The listing builds one solid part. Answer for the finished solid, in the listing's coordinates (mm). A direction names the side the tool comes from. Round coordinates to 2 decimals unless told otherwise and drop trailing zeros. Loops run counter-clockwise (first coordinate to the right, second up) from the corner with the lowest first, then second, coordinate; pieces in that order, holes last. Notation, with made-up numbers: (81, 66.25) -> (136, 66.25) arc R30 ccw to (136, 88.25) -> close; hole circle Ø9 at (-26.75, 70.25). An arc over 180 degrees is marked (long way). Answer in a Markdown table with one row per item. Add a question column.
Autodesk Inventor part; units mm, degrees
ref_plane "YZ Plane" through (0, 0, 0) normal (1, 0, 0) x (0, 1, 0)
ref_plane "XZ Plane" through (0, 0, 0) normal (0, 1, 0) x (-1, 0, 0)
ref_plane "XY Plane" through (0, 0, 0) normal (0, 0, 1) x (1, 0, 0)
sketch "Sketch1" plane through (0, 0, 0) normal (0, 0, 1) x (1, 0, 0)
  line L0 (-85, 50) -> (85, 50)
  line L1 (85, 50) -> (85, -50)
  line L2 (85, -50) -> (-85, -50)
  line L3 (-85, -50) -> (-85, 50)
  line L4 (-85, 50) -> (85, -50) construction
  line L5 (85, 50) -> (-85, -50) construction
  point P0 (0, 0)
  dimension "d0" = 170
  dimension "d1" = 100
extrude "Extrusion1" add sketch "Sketch1" along normal mid plane 10
sketch "Sketch2" plane through (0, 0, 5) normal (0, 0, 1) x (1, 0, 0)
  line L0 (-70, 35) -> (70, 35)
  line L1 (70, 35) -> (70, -35)
  line L2 (70, -35) -> (-70, -35)
  line L3 (-70, -35) -> (-70, 35)
  line L4 (-70, 35) -> (70, -35) construction
  line L5 (70, 35) -> (-70, -35) construction
  point P0 (0, 0)
  dimension "d4" = 140
  dimension "d5" = 70
extrude "Extrusion2" cut sketch "Sketch2" against normal blind 10
sketch "Sketch4" plane through (0, 0, 5) normal (0, 0, 1) x (1, 0, 0)
  line L0 (-85, 50) -> (-85, -50)
  line L1 (85, 50) -> (-85, 50)
  line L2 (-85, -50) -> (85, -50)
  line L3 (85, -50) -> (85, 50)
  point P0 (0, 0)
  point P1 (-80, 0)
  point P2 (-80, -45)
  point P3 (0, -45)
  point P4 (-55, -45)
  point P5 (55, -45)
  point P6 (80, -45)
  point P7 (80, 0)
  point P8 (-80, 45)
  point P9 (-55, 45)
  point P10 (55, 45)
  point P11 (0, 45)
  point P12 (80, 45)
  dimension "d72" = 50
  dimension "d73" = 5
  dimension "d74" = 5
  dimension "d75" = 85
  dimension "d78" = 25
  dimension "d80" = 5
  dimension "d81" = 5
  dimension "d82" = 25
  dimension "d85" = 160
  dimension "d115" = 5
  dimension "d116" = 5
  dimension "d117" = 5
  dimension "d120" = 90
  dimension "d125" = 45
hole "Hole2" at (-80, 0, 5) at (-80, -45, 5) at (0, -45, 5) at (-55, -45, 5) at (55, -45, 5) at (80, -45, 5) at (80, 0, 5) at (80, 45, 5) at (55, 45, 5) at (0, 45, 5) at (-55, 45, 5) at (-80, 45, 5) direction (0, 0, -1) diameter 4.3688 end through all
properties part number "gasket"
Item 1: Section C-C, the plane y = 0 is taken. Write down the section's boundary in (x, z), and give its area (3 significant figures).
Item 2: The mould has two halves that part along Y. Classify faces 1 (the flat face through (-70, 0, 0)), 2 (the flat face through (-1, 50, 0)), 3 (the flat face through (0, -37, 5)): +Y half, -Y half, draft (parallel to the pull), parting line (faces both ways), or undercut.
Item 3: For faces 4 (the flat face through (0, -37, -5)), 5 (the flat face through (1, -35, 0)), determine the directions among +Z, -Z, +X, -X, +Y, -Y from which every point of the face is accessible in a straight line to the end or side of a thin tool.
Item 4: Section A-A, the plane x = 80 is taken. Write down the section's boundary in (y, z), and give its area (3 significant figures).
Item 5: Section B-B, the plane y = 45 is taken. Write down the section's boundary in (x, z), and give its area (3 significant figures).
Item 6: Consider L1, parallel to Y at x = 0, z = -2.25; L2, parallel to X at y = 0, z = 2; L3, parallel to X at y = 45, z = 0. Determine where each line is inside the solid, lowest interval first. Write a range as from..to.
Item 7: Section D-D, the plane x = -20.5 is taken. Write down the section's boundary in (y, z).
Here are the results:
| question | item | result |
|---|---|---|
| 1 | outline | (-85, -5) -> (-82.18, -5) -> (-82.18, 5) -> (-85, 5) -> close; (-77.82, -5) -> (-70, -5) -> (-70, 5) -> (-77.82, 5) -> close; (70, -5) -> (77.82, -5) -> (77.82, 5) -> (70, 5) -> close; (82.18, -5) -> (85, -5) -> (85, 5) -> (82.18, 5) -> close |
| 1 | area | 213 mm² |
| 2 | face 1 | undercut |
| 2 | face 2 | +Y half |
| 2 | face 3 | draft |
| 3 | face 4 | -Z, +X, -X, +Y, -Y |
| 3 | face 5 | +Z, -Z |
| 4 | outline | (-50, -5) -> (-47.18, -5) -> (-47.18, 5) -> (-50, 5) -> close; (-42.82, -5) -> (-2.18, -5) -> (-2.18, 5) -> (-42.82, 5) -> close; (2.18, -5) -> (42.82, -5) -> (42.82, 5) -> (2.18, 5) -> close; (47.18, -5) -> (50, -5) -> (50, 5) -> (47.18, 5) -> close |
| 4 | area | 869 mm² |
| 5 | outline | (-85, -5) -> (-82.18, -5) -> (-82.18, 5) -> (-85, 5) -> close; (-77.82, -5) -> (-57.18, -5) -> (-57.18, 5) -> (-77.82, 5) -> close; (-52.82, -5) -> (-2.18, -5) -> (-2.18, 5) -> (-52.82, 5) -> close; (2.18, -5) -> (52.82, -5) -> (52.82, 5) -> (2.18, 5) -> close; (57.18, -5) -> (77.82, -5) -> (77.82, 5) -> (57.18, 5) -> close; (82.18, -5) -> (85, -5) -> (85, 5) -> (82.18, 5) -> close |
| 5 | area | 1,480 mm² |
| 6 | L1 | y = -50..-47.18, -42.82..-35, 35..42.82, 47.18..50 |
| 6 | L2 | x = -85..-82.18, -77.82..-70, 70..77.82, 82.18..85 |
| 6 | L3 | x = -85..-82.18, -77.82..-57.18, -52.82..-2.18, 2.18..52.82, 57.18..77.82, 82.18..85 |
| 7 | outline | (-50, -5) -> (-35, -5) -> (-35, 5) -> (-50, 5) -> close; (35, -5) -> (50, -5) -> (50, 5) -> (35, 5) -> close |
